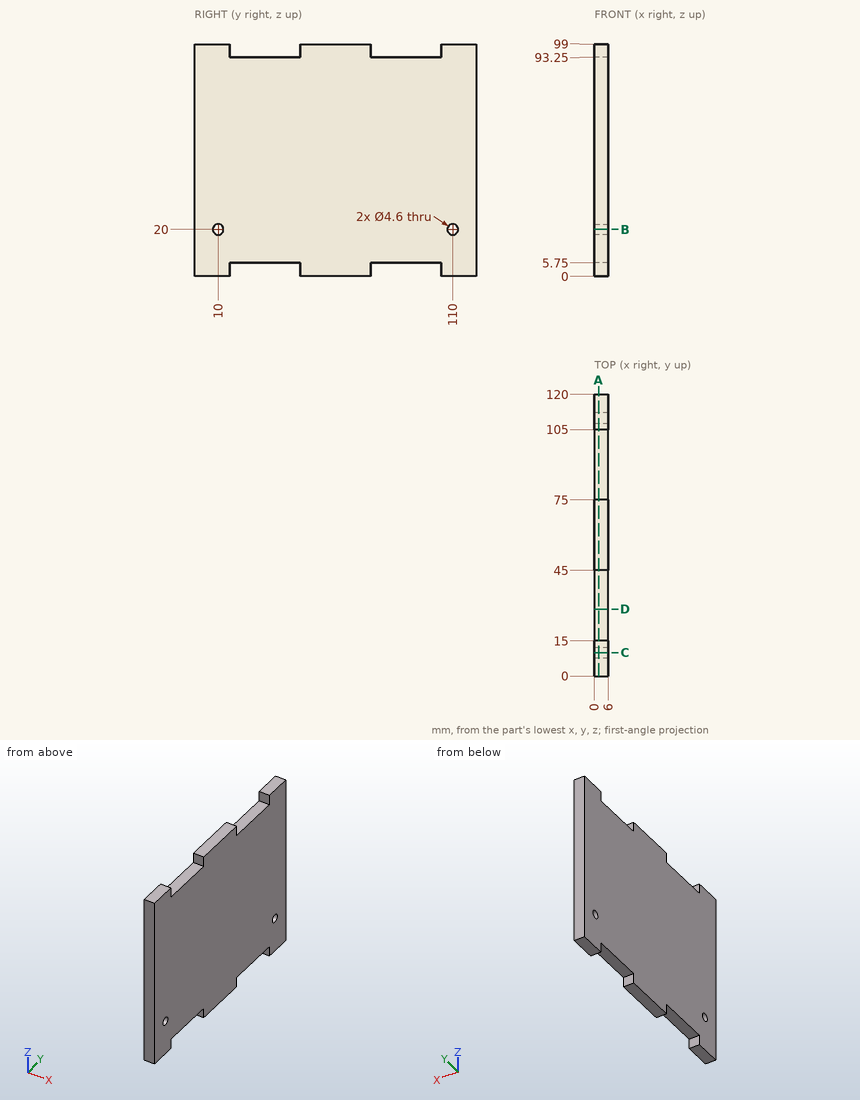
Verification items for this drawing (mm, ordinates from the low corner). Coordinates: 2 decimals unless noted, no trailing zeros. Order: outer loops, then holes, each group sorted by start corner. A loop starts at its lowest first (then second) coordinate and runs counter-clockwise, first axis right, second up. Notation, with made-up numbers: (6.5, 47) - (16.5, 47) arc R19 ccw to (16.5, 74) - close; hole circle Ø7 at (-2, -34.75). An arc over 180 degrees is marked (long way). Use one line per item in the form item = value.
1. Section check C-C (y = 10). Record the boundary of the cut face in (x, z).
Here are the results:
outline = (0, 0) - (6, 0) - (6, 17.7) - (0, 17.7) - close; (0, 22.3) - (6, 22.3) - (6, 99) - (0, 99) - close
2. Section check B-B (z = 20). Record the boundary of the cut face in (x, y).
Here are the results:
outline = (0, 0) - (6, 0) - (6, 7.7) - (0, 7.7) - close; (0, 12.3) - (6, 12.3) - (6, 107.7) - (0, 107.7) - close; (0, 112.3) - (6, 112.3) - (6, 120) - (0, 120) - close
3. Section check A-A (x = 1.9). Record the boundary of the cut face in (y, z), then the cut area to 3 significant figures.
Here are the results:
outline = (0, 0) - (15, 0) - (15, 5.75) - (45, 5.75) - (45, 0) - (75, 0) - (75, 5.75) - (105, 5.75) - (105, 0) - (120, 0) - (120, 99) - (105, 99) - (105, 93.25) - (75, 93.25) - (75, 99) - (45, 99) - (45, 93.25) - (15, 93.25) - (15, 99) - (0, 99) - close; hole circle Ø4.6 at (10, 20); hole circle Ø4.6 at (110, 20)
area = 11,200 mm²
4. Section check D-D (y = 28.5). Record the boundary of the cut face in (x, z).
Here are the results:
outline = (0, 5.75) - (6, 5.75) - (6, 93.25) - (0, 93.25) - close
5. Gauge pin test, flat ends, axial feed: pin 1 (3 mm diameter, centred on y = 110, z = 20, fed in from -X); pin 2 (6 mm diameter, centred on y = 10, z = 20, fed in from -X); pin 3 (3 mm diameter, centred on x = 2.5, y = 96, fed in from -Z). Record the tip position at first contact, or that the pin passes through.
Here are the results:
pin_1 = through
pin_2 = 0
pin_3 = 5.75
6. Scan lines: line 1 (Y direction, x = 1.75, z = 20); line 2 (Y direction, x = 5.5, z = 94); line 3 (Z direction, x = 0.95, y = 77). Record each from-to range of solid material in increasing order.
Here are the results:
line_1 = 0 to 7.7, 12.3 to 107.7, 112.3 to 120
line_2 = 0 to 15, 45 to 75, 105 to 120
line_3 = 5.75 to 93.25
